Design review of the part built by this model. Coordinates are the model's own, in mm. A direction names the side the tool comes from. Give positions to 0.01 mm unless a question says otherwise; leave off trailing zeros. Order: outer loops, then holes, each group sorted by start corner. A loop starts at its lowest first (then second) coordinate and runs counter-clockwise, first axis right, second up. Notation, with made-up numbers: (-34.5, 71.25) -> (-5.5, 71.25) arc R19 cw to (-5.5, 83.25) -> close; hole circle Ø3 at (30, 39.25). An arc over 180 degrees is marked (long way). Return JSON: item names as keys, results as strings.
```python
from build123d import *

# Parameters (mm, degrees)
F1_DEPTH = 150


# Not quite as in the source:
# - a feature of the source that left no trace in its solid (it failed there, or was rolled back) is left out


with BuildPart() as f1:
    # F0 (on Front) → F1 (new body)
    with BuildSketch(Plane.XZ):
        Polygon((0.316192396, 10.0656654686), (-12.7883255482, 10.0656654686), (-12.7883255482, -5.258587189), (0.2559647712, -5.1627713866), (12.8449704498, -5.0702998415), (12.8449704498, 10.0656654686), align=None)
        Polygon((0.316192396, 18.6481969431), (-12.7883255482, 10.0656654686), (0.316192396, 10.0656654686), align=None)
        Polygon((12.8449704498, -5.0702998415), (0.2559647712, -5.1627713866), (0.316192396, -13.3621143177), align=None)
    extrude(amount=F1_DEPTH)


solid = f1.part
```
Item 1: Add section B-B (x = 6.75). Give the boundary of the cut face in (y, z), plus the area to 3 significant figures.
Result set:
{"outline": "(-150, -9.1) -> (0, -9.1) -> (0, 10.07) -> (-150, 10.07) -> close", "area": "2,880 mm^2"}
Item 2: For pin 1 (3 mm diameter, centred on x = 2, y = -133, fed in from +Z); pin 2 (1 mm diameter, centred on x = -7.5, y = -92, fed in from +Z); pin 3 (1.5 mm diameter, centred on x = 0, y = -76, fed in from +Z), all flat-tipped, find the tip position at first contact; note any pin that passes through.
Result set:
{"pin 1": "stops at z = 10.07", "pin 2": "stops at z = 13.86", "pin 3": "stops at z = 18.65"}
Item 3: Add section C-C (z = -11). Give the boundary of the cut face in (x, y).
Result set:
{"outline": "(0.3, -150) -> (3.89, -150) -> (3.89, 0) -> (0.3, 0) -> close"}
Item 4: Add section A-A (y = -26). Give the boundary of the cut face in (x, z).
Result set:
{"outline": "(-12.79, -5.26) -> (0.26, -5.16) -> (0.32, -13.36) -> (12.84, -5.07) -> (12.84, 10.07) -> (0.32, 10.07) -> (0.32, 18.65) -> (-12.79, 10.07) -> close"}
Item 5: Machinability: for faces 1 (the face through (0, 0, 3)), 2 (the face through (7, -74, 10.066)), which of the approach directions +Z, -Z, +X, -X, +Y, -Y give a long, thin tool a straight path to every point of the face, cutting with its end or side? Answer none if there is none.
Result set:
{"face 1": "+Z, -Z, +X, -X, +Y", "face 2": "+Z, +X, +Y, -Y"}
Item 6: Wall thickness on L1, parallel to Z at x = 11.25, y = -64; L2, parallel to Z at x = -0.5, y = -90.5; L3, parallel to X at y = -81, z = -11: over which ranges is each line inside the solid? List them lowest first. Write a range as [from, to].
Result set:
{"L1": "z = [-6.13, 10.07]", "L2": "z = [-5.17, 18.11]", "L3": "x = [0.3, 3.89]"}
